The figure shows three views and two pictorial views of one solid part (mm, origin at its lowest corner). Answer the questions. Coordinates: 2 decimals unless noted, no trailing zeros. Write each loop counter-clockwise with the first axis right and the second up, starting at its lowest first coordinate (ties: lowest second). Pieces come first, ordered by that corner, then holes.
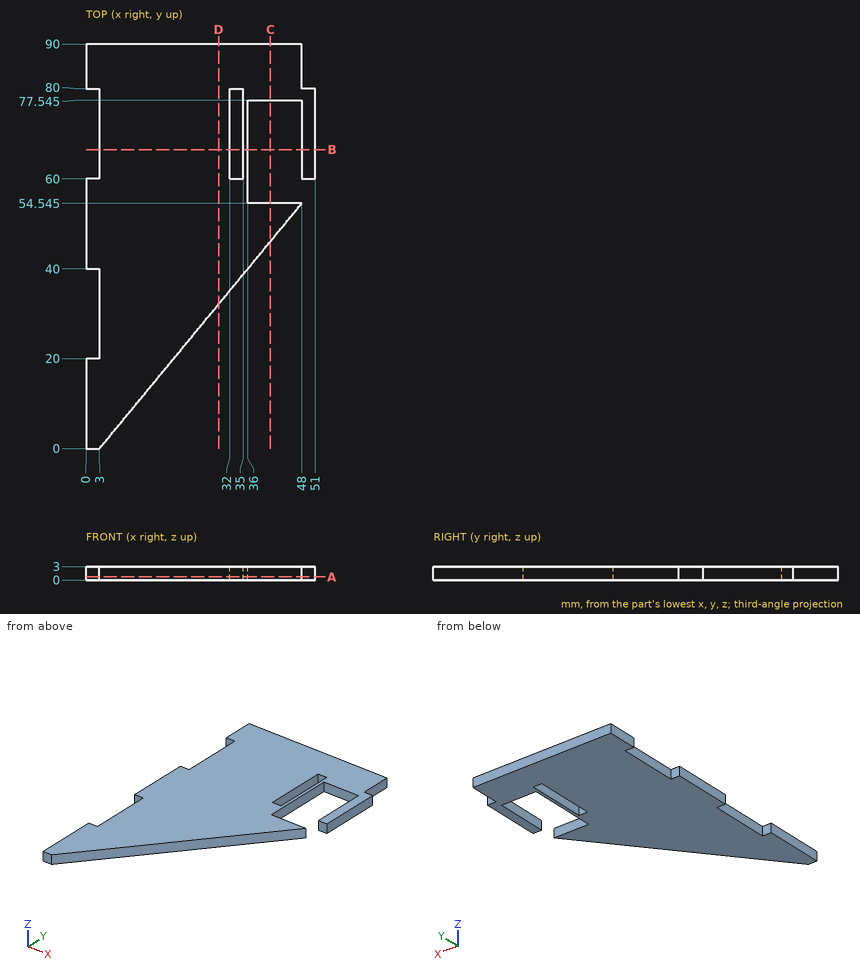
Q1. The part is cut by section C-C, the plane x = 41. Write down the section's boundary in (y, z) (1 decimal).
Answers below:
outline: (46.1, 0) - (54.5, 0) - (54.5, 3) - (46.1, 3) - close; (77.5, 0) - (90, 0) - (90, 3) - (77.5, 3) - close
Q2. Find the intervals of material crossed by probe 1 along X at (y, z) = (75, 0.35); probe 2 along X at (y, z) = (83, 2.85); probe 3 along Y at (x, z) = (44.5, 0.2) (1 decimal), in increasing order.
Answers below:
probe 1: x = 3 to 32, 35 to 36, 48 to 51
probe 2: x = 0 to 48
probe 3: y = 50.3 to 54.5, 77.5 to 90
Q3. The part is cut by section D-D, the plane x = 29.5. Write down the section's boundary in (y, z).
Answers below:
outline: (32.12, 0) - (90, 0) - (90, 3) - (32.12, 3) - close
Q4. The part is cut by section A-A, the plane z = 0.75. Write down the section's boundary in (x, y) (1 decimal).
Answers below:
outline: (0, 0) - (3, 0) - (48, 54.5) - (36, 54.5) - (36, 77.5) - (48, 77.5) - (48, 60) - (51, 60) - (51, 80) - (48, 80) - (48, 90) - (0, 90) - (0, 80) - (3, 80) - (3, 60) - (0, 60) - (0, 40) - (3, 40) - (3, 20) - (0, 20) - close; hole (32, 60) - (35, 60) - (35, 80) - (32, 80) - close
Q5. The part is cut by section B-B, the plane y = 66.5. Write down the section's boundary in (x, z).
Answers below:
outline: (3, 0) - (32, 0) - (32, 3) - (3, 3) - close; (35, 0) - (36, 0) - (36, 3) - (35, 3) - close; (48, 0) - (51, 0) - (51, 3) - (48, 3) - close
Q6. Given pin 1 (1.5 mm diameter, centred on x = 33.5, z = 1.5, fed in from -Y); pin 2 (1.5 mm diameter, centred on x = 49, z = 2, fed in from +Y); pin 3 (1.5 mm diameter, centred on y = 82.5, z = 1.5, fed in from +X), each flat-ended and moving along its own axis, determine where each tip first touches the part or whether it passes through.
Answers below:
pin 1: stops at y = 36.06
pin 2: stops at y = 80
pin 3: stops at x = 48
